Part model, mm, in its own coordinate system. Face numbers are marked on the shaded views. A direction names the side the tool comes from. Give positions to 0.01 mm unless a question says otherwise; leave off trailing zeros. Order: outer loops, then holes, each group sorted by start corner. A loop starts at its lowest first (then second) coordinate and runs counter-clockwise, first axis right, second up. Notation, with made-up numbers: (30.5, 27.5) - (54.5, 27.5) arc R22 cw to (54.5, 53.5) - close; hole circle Ø2 at (-37, 89.5). An arc over 180 degrees is marked (long way). One line per item, written item: value.
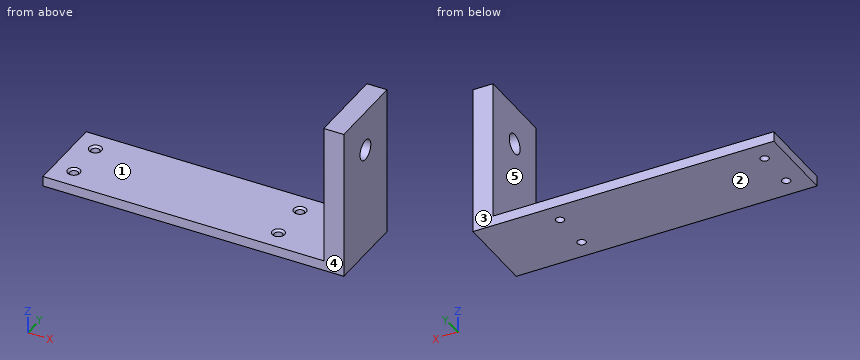
Solid Edge part; units mm, degrees
sketch "Sketch1" plane through (0, 0, 0) normal (0, 0, 1) x (1, 0, 0)
  line L0 (150, 0) -> (150, 40)
  line L1 (150, 40) -> (0, 40)
  line L2 (0, 40) -> (0, 0)
  line L3 (0, 0) -> (150, 0)
extrude "Protrusion1" add sketch "Sketch1" along normal blind 5
sketch "Sketch2" plane through (75, 20, 5) normal (0, 0, 1) x (1, 0, 0)
  line L0 (65, 20) -> (75, 20)
  line L1 (75, 20) -> (75, -20)
  line L2 (75, -20) -> (65, -20)
  line L3 (65, -20) -> (65, 20)
extrude "Extrusionsausprägung_2" add sketch "Sketch2" along normal blind 70
hole "Bohrung_1" at (10, 30, 5) direction (0, 0, -1) diameter 4.2 end up to next start chamfer 1 start chamfer angle 45
hole "Hole1" at (10, 10, 5) direction (0, 0, -1) diameter 4.2 end up to next start chamfer 1 start chamfer angle 45
hole "Hole2" at (112, 10, 5) direction (0, 0, -1) diameter 4.2 end up to next start chamfer 1 start chamfer angle 45
hole "Hole3" at (112, 30, 5) direction (0, 0, -1) diameter 4.2 end up to next start chamfer 1 start chamfer angle 45
hole "Bohrung_6" at (150, 20, 55) direction (-1, 0, 0) diameter 10 end up to next
1) Wall check: line 1 along X through (y, z) = (10, 2.4); line 2 along Y through (x, z) = (10, 2.65); line 3 along Z through (x, y) = (47, 5). Give the ranges that are in metal, low to high. Write a range as [from, to].
Answer:
line 1: x = [0, 7.9], [12.1, 109.9], [114.1, 150]
line 2: y = [0, 7.9], [12.1, 27.9], [32.1, 40]
line 3: z = [0, 5]
2) Slice it at B-B on y = 10. Write the cut outline in (x, z), then the cut area to 3 significant figures.
Answer:
outline: (0, 0) - (7.9, 0) - (7.9, 4) - (6.9, 5) - (0, 5) - close; (12.1, 0) - (109.9, 0) - (109.9, 4) - (108.9, 5) - (13.1, 5) - (12.1, 4) - close; (114.1, 0) - (150, 0) - (150, 75) - (140, 75) - (140, 5) - (115.1, 5) - (114.1, 4) - close
area: 1,410 mm2
3) Slice it at A-A on z = 55. Write the cut outline in (x, y), then the cut area to 3 significant figures.
Answer:
outline: (140, 0) - (150, 0) - (150, 15) - (140, 15) - close; (140, 25) - (150, 25) - (150, 40) - (140, 40) - close
area: 300 mm2
4) Drop flat-ended pins along their axis: P1, Ø12, axis at y = 20.5, z = 37, coming from the -X side; P2, Ø5, axis at x = 96.5, y = 14, coming from the +Z side; P3, Ø1.5, axis at x = 17, y = 34, coming from the -Z side. Give the stop position or say it passes through.
Answer:
P1: stops at x = 140
P2: stops at z = 5
P3: stops at z = 0
5) Slice it at C-C on x = 10. Write the cut outline in (y, z).
Answer:
outline: (0, 0) - (7.9, 0) - (7.9, 4) - (6.9, 5) - (0, 5) - close; (12.1, 0) - (27.9, 0) - (27.9, 4) - (26.9, 5) - (13.1, 5) - (12.1, 4) - close; (32.1, 0) - (40, 0) - (40, 5) - (33.1, 5) - (32.1, 4) - close
6) Two-plate mould, pull along Z, no slides. Class the marked faces 1, 2 and 3: pulls with the +Z half, pulls with the -Z half, needs draft (parallel to the pull), parting line crosses it, or undercut.
Answer:
face 1: pulls with the +Z half
face 2: pulls with the -Z half
face 3: needs draft
7) Slice it at D-D on y = 20. Write the cut outline in (x, z), then the cut area to 3 significant figures.
Answer:
outline: (0, 0) - (150, 0) - (150, 50) - (140, 50) - (140, 5) - (0, 5) - close; (140, 60) - (150, 60) - (150, 75) - (140, 75) - close
area: 1,350 mm2
8) Which spindle directions (+Z, -Z, +X, -X, +Y, -Y) get a long thin tool onto all of the face, cutting with end or side? Do the marked faces 4 and 5. Say none if no direction does.
Answer:
face 4: +Z, -Z, +X, -X, -Y
face 5: +Z, -X, +Y, -Y
